Geometry check sheet. Reference: the model listing, model coordinates, mm. Face numbers are marked on the shaded views. A direction names the side the tool comes from. Round coordinates to 2 decimals unless told otherwise and drop trailing zeros. Write each loop counter-clockwise with the first axis right and the second up, starting at its lowest first coordinate (ties: lowest second). Pieces come first, ordered by that corner, then holes. Notation, with made-up numbers: (73, 2) -> (112, 2) arc R24 cw to (112, 18) -> close; hole circle Ø11 at (-36.5, -15.75). An arc over 180 degrees is marked (long way). Use a Markdown table: item, result.
Autodesk Inventor part; units mm, degrees
ref_plane "XZ Plane" through (0, 0, 0) normal (0, 1, 0) x (-1, 0, 0)
ref_plane "XY Plane" through (0, 0, 0) normal (0, 0, 1) x (1, 0, 0)
sketch "Sketch1" plane through (0, 0, 0) normal (0, 1, 0) x (-1, 0, 0)
  line L0 (3.175, 0) -> (111.125, 0)
  line L1 (114.3, 3.175) -> (114.3, 26.9875)
  line L2 (111.125, 30.1625) -> (92.075, 30.1625)
  line L3 (92.075, 84.1375) -> (111.125, 84.1375)
  line L4 (114.3, 87.3125) -> (114.3, 111.125)
  line L5 (111.125, 114.3) -> (3.175, 114.3)
  line L6 (0, 111.125) -> (0, 87.3125)
  line L7 (3.175, 84.1375) -> (22.225, 84.1375)
  line L8 (22.225, 30.1625) -> (3.175, 30.1625)
  line L9 (0, 3.175) -> (0, 26.9875)
  arc A0 (114.3, 111.125) -> (111.125, 114.3) centre (111.125, 111.125) ccw
  arc A1 (111.125, 84.1375) -> (114.3, 87.3125) centre (111.125, 87.3125) ccw
  arc A2 (114.3, 26.9875) -> (111.125, 30.1625) centre (111.125, 26.9875) ccw
  arc A3 (111.125, 0) -> (114.3, 3.175) centre (111.125, 3.175) ccw
  arc A4 (0, 3.175) -> (3.175, 0) centre (3.175, 3.175) ccw
  arc A5 (3.175, 30.1625) -> (0, 26.9875) centre (3.175, 26.9875) ccw
  arc A6 (0, 87.3125) -> (3.175, 84.1375) centre (3.175, 87.3125) ccw
  arc A7 (3.175, 114.3) -> (0, 111.125) centre (3.175, 111.125) ccw
  line L10 (92.075, 84.1375) -> (22.225, 84.1375)
  line L11 (92.075, 30.1625) -> (22.225, 30.1625)
  point P0 (0, 0)
  point P1 (114.3, 0)
  point P2 (114.3, 30.1625)
  point P3 (88.9, 30.1625)
  point P4 (88.9, 84.1375)
  point P5 (114.3, 84.1375)
  point P6 (114.3, 114.3)
  point P7 (0, 114.3)
  point P8 (0, 84.1375)
  point P9 (25.4, 84.1375)
  point P10 (25.4, 30.1625)
  point P11 (0, 30.1625)
  dimension "d0" = 114.3
  dimension "d1" = 30.1625
  dimension "d2" = 25.4
  dimension "d4" = 30.1625
  dimension "d5" = 114.3
  dimension "d6" = 25.4
  dimension "d9" = 3.175
  dimension "d42" = 114.3
extrude "Extrusion1" add sketch "Sketch1" along normal blind 1.5875
ref_plane "Work Plane1" through (-25.4, 0, 0) normal (1, 0, 0) x (0, 1, 0)
sketch "Sketch3" plane through (-25.4, 0, 0) normal (1, 0, 0) x (0, 1, 0)
  line L0 (0, 84.1375) -> (1.5875, 84.1375)
  line L1 (0.7937, 84.1375) -> (1.8521, 81.1441)
  line L2 (0.7937, 84.1375) -> (3.9688, 84.1375) construction
  line L3 (0, 30.1625) -> (1.5875, 30.1625) construction
  line L4 (7.9375, 57.15) -> (-6.35, 57.15) construction
  line L5 (1.8521, 81.1441) -> (1.8521, 57.15)
  line L6 (0.7938, 30.1625) -> (1.8521, 33.1559)
  line L7 (1.8521, 33.1559) -> (1.8521, 57.15)
  line L8 (0.5015, 30.2658) -> (1.5421, 33.2091)
  line L9 (1.5421, 33.2091) -> (1.5421, 55.5625)
  line L10 (1.5421, 55.5625) -> (1.5421, 81.0909)
  line L11 (1.5421, 81.0909) -> (0.3554, 84.4475)
  line L12 (0.3554, 84.4475) -> (3.9687, 84.4475)
  line L13 (0.5015, 30.2658) -> (0.465, 30.1625)
  line L14 (0.7938, 30.1625) -> (0.465, 30.1625)
  line L15 (0.7937, 84.1375) -> (0.465, 84.1375)
  point P0 (0, 0)
  dimension "d11" = 3.175
  dimension "d12" = 70.529
extrude "Extrusion2" add sketch "Sketch3" against normal blind 63.5
sketch "Sketch4" plane through (0, 1.5875, 0) normal (0, 1, 0) x (1, 0, 0)
  circle A0 centre (-107.95, -6.35) radius 1.5875
  line L0 (-111.125, -30.1625) -> (-3.175, -30.1625)
  line L1 (-114.3, -3.175) -> (-114.3, -26.9875)
  circle A1 centre (-6.35, -6.35) radius 1.5875
  circle A2 centre (-107.95, -107.95) radius 1.5875
  circle A3 centre (-6.35, -107.95) radius 1.5875
  line L2 (-3.175, 0) -> (-111.125, 0)
  line L3 (-111.125, -114.3) -> (-3.175, -114.3)
  line L4 (-107.95, -6.35) -> (-76.5191, -6.35) construction
  line L5 (-107.95, -6.35) -> (-82.55, -6.35) construction
  circle A4 centre (-95.25, -19.05) radius 1.5875
  circle A5 centre (-20.6375, -19.05) radius 1.5875
  circle A6 centre (-95.25, -93.6625) radius 1.5875
  circle A7 centre (-20.6375, -93.6625) radius 1.5875
  line L6 (0, -26.9875) -> (0, -3.175)
  point P0 (0, 0)
  point P1 (-114.3, -15.0812)
  dimension "d15" = 3.175
  dimension "d17" = 6.35
  dimension "d28" = 101.6
  dimension "d31" = 101.6
  dimension "d43" = 107.95
  dimension "d48" = 3.175
  dimension "d51" = 74.6125
  dimension "d54" = 74.6125
  dimension "d57" = 95.25
  dimension "d58" = 95.25
extrude "Extrusion4" cut sketch "Sketch4" against normal blind 63.5
properties part number "Monitor Base v1.0"
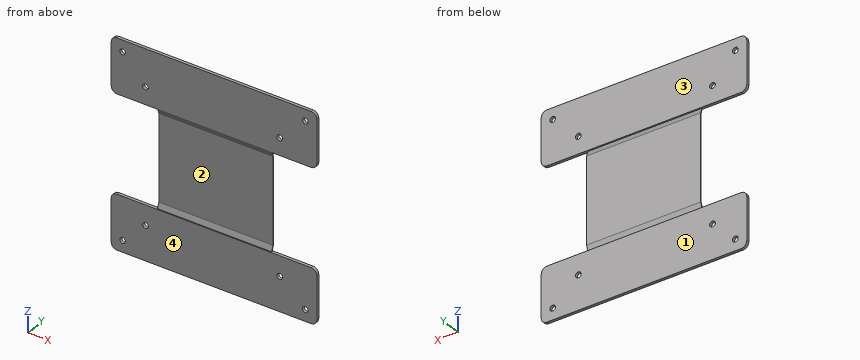
(1) Section check B-B on x = -95.25. State how many separate pieces and enclosed holes the cut face has, plus the area to 3 significant figures.
A:
| item | result |
|---|---|
| separate pieces | 4 |
| enclosed holes | 0 |
| area | 85.7 mm2 |
(2) Section check D-D on z = 100.5. Record the cut outline in (x, y).
A:
| item | result |
|---|---|
| outline | (-114.3, 0) -> (0, 0) -> (0, 1.59) -> (-114.3, 1.59) -> close |
(3) Access from +Z, -Z, +X, -X, +Y, -Y to the whole of each face (thin tool, end or side, straight path). Record for the marked faces 3 and 4.
A:
| item | result |
|---|---|
| face 3 | +Z, +X, -X, +Y |
| face 4 | +Z, -Z, +X, -X, -Y |
(4) Release check for a two-part mould opening along Z. For the marked faces 1 and 2 record: +Z half, -Z half, draft (parallel to the pull), parting line (faces both ways), or undercut.
A:
| item | result |
|---|---|
| face 1 | draft |
| face 2 | undercut |
(5) Section check A-A on z = 6.35. Record the cut outline in (x, y), plus the area to 3 significant figures.
A:
| item | result |
|---|---|
| outline | (-114.3, 0) -> (-109.54, 0) -> (-109.54, 1.59) -> (-114.3, 1.59) -> close; (-106.36, 0) -> (-7.94, 0) -> (-7.94, 1.59) -> (-106.36, 1.59) -> close; (-4.76, 0) -> (0, 0) -> (0, 1.59) -> (-4.76, 1.59) -> close |
| area | 171 mm2 |
(6) Gauge pin test, flat ends, axial feed: pin 1 Ø1.9 at (x, z) = (-20.64, 19.05) entering from +Y (1 decimal); pin 2 Ø4 at (x, z) = (-107.95, 107.95) entering from +Y; pin 3 Ø1.1 at (y, z) = (1.5, 53) entering from -X; pin 4 Ø14.5 at (x, z) = (-66.5, 55.5) entering from -Y. Record the tip position at first contact, or that the pin passes through.
A:
| item | result |
|---|---|
| pin 1 | passes through |
| pin 2 | stops at y = 1.59 |
| pin 3 | stops at x = -88.9 |
| pin 4 | stops at y = 1.54 |
(7) Thickness scan on line 1 (Z direction, x = -107.95, y = 1); line 2 (Z direction, x = -11, y = 0.85); line 3 (X direction, y = 1.05, z = 6.35). Record the ranges inside material, lowest first.
A:
| item | result |
|---|---|
| line 1 | z = 0 to 4.76, 7.94 to 30.16, 84.14 to 106.36, 109.54 to 114.3 |
| line 2 | z = 0 to 30.16, 84.14 to 114.3 |
| line 3 | x = -114.3 to -109.54, -106.36 to -7.94, -4.76 to 0 |
